from build123d import *

# Parameters (mm, degrees)
F0_W     = 19.05
F0_H     = 19.05
F1_DEPTH = 19.05
F2_DEPTH = 19.05
F3_W     = 19.05
F3_H     = 19.05
F4_DEPTH = 19.05
F5_W     = 19.05
F5_H     = 19.05
F6_DEPTH = 19.05


with BuildPart() as f1:
    # F0 (on Top) → F1 (new body)
    with BuildSketch(Plane.XY):
        with Locations((9.525, 9.525)):
            Rectangle(F0_W, F0_H)
    extrude(amount=F1_DEPTH)

    # F2 (add): a face of the model
    f2_faces = [f1.faces().sort_by_distance(p)[0] for p in [
        (9.525, 9.525, 19.05),
    ]]
    extrude(f2_faces, amount=F2_DEPTH)

    # F3 (on face) → F4 (join)
    with BuildSketch(Plane(origin=(0, 19.05, 0), x_dir=(-1, 0, 0), z_dir=(0, 1, 0))):
        with Locations((-9.525, 28.575)):
            Rectangle(F3_W, F3_H)
    extrude(amount=F4_DEPTH)

    # F5 (on face) → F6 (join)
    with BuildSketch(Plane.XY.offset(38.1)):
        with Locations((9.525, 9.525)):
            Rectangle(F5_W, F5_H)
    extrude(amount=F6_DEPTH)


solid = f1.part
Here's how the part is built. I have some questions about the finished solid (model axes, mm). A direction names the side the tool comes from. Give positions to 0.01 mm unless a question says otherwise; leave off trailing zeros. Loops run counter-clockwise (first coordinate to the right, second up) from the corner with the lowest first, then second, coordinate; pieces in that order, holes last. Notation, with made-up numbers: (-2.75, 39.5) -> (53.25, 39.5) arc R28 ccw to (53.25, 68.5) -> close; hole circle Ø9 at (68.5, -28.75). An arc over 180 degrees is marked (long way). Answer as a JSON object with one key per item and string values. Group by question number.
Item 1: On a 3-axis mill with a long thin cutter (end or side, diameter ignored), from which of +Z, -Z, +X, -X, +Y, -Y can I reach the whole of each face in a straight line? I mean faces 1 (the flat face through (9, 10, 57.15)), 2 (the flat face through (9, 19.05, 47)), 3 (the flat face through (9, 19.05, 9)). Say none if no direction works.
Item 2: Imagine slicing it at A-A on x = 11. Write out the boundary of the cut face in (y, z), then the cut area to 3 significant figures.
Item 3: I need wall thicknesses on L1, parallel to Y at x = 7.5, z = 39; L2, parallel to Z at x = 14, y = 21. Which ranges of each line are inside material? Lowest first, please.
Item 4: Imagine slicing it at B-B on y = 25. Write out the boundary of the cut face in (x, z).
Item 5: Imagine slicing it at C-C on z = 17.5. Write out the boundary of the cut face in (x, y).
Item 6: Will these pins go through, and if not, where does the flat tip stop? pin 1 (9.5 mm diameter, centred on x = 12, z = 9, fed in from +Y); pin 2 (5.5 mm diameter, centred on x = 10, y = 29, fed in from -Z); pin 3 (10 mm diameter, centred on x = 7, y = 34, fed in from +Z).
Answer list:
{
 "1": {"face 1": "+Z, +X, -X, +Y, -Y", "face 2": "+Z, +X, -X, +Y", "face 3": "-Z, +X, -X, +Y"},
 "2": {"outline": "(0, 0) -> (19.05, 0) -> (19.05, 19.05) -> (38.1, 19.05) -> (38.1, 38.1) -> (19.05, 38.1) -> (19.05, 57.15) -> (0, 57.15) -> close", "area": "1,450 mm2"},
 "3": {"L1": "y = 0 to 19.05", "L2": "z = 19.05 to 38.1"},
 "4": {"outline": "(0, 19.05) -> (19.05, 19.05) -> (19.05, 38.1) -> (0, 38.1) -> close"},
 "5": {"outline": "(0, 0) -> (19.05, 0) -> (19.05, 19.05) -> (0, 19.05) -> close"},
 "6": {"pin 1": "stops at y = 19.05", "pin 2": "stops at z = 19.05", "pin 3": "stops at z = 38.1"}
}
